The listing builds one solid part. Answer for the finished solid, in the listing's coordinates (mm). A direction names the side the tool comes from. Round coordinates to 2 decimals unless told otherwise and drop trailing zeros. Write each loop counter-clockwise with the first axis right and the second up, starting at its lowest first coordinate (ties: lowest second). Pieces come first, ordered by that corner, then holes. Notation, with made-up numbers: M 27,-12 L 48,-12 A24 cw 48,26 Z; hole C 5,68.25 d5. An arc over 180 degrees is marked long. Put each result on its own line as item: value. Start each with the question number.
```python
from build123d import *

# Parameters (mm, degrees)
F0_R     = 6.35
F1_DEPTH = 50.8
F2_R     = 44.45
F3_DEPTH = 127
F4_R     = 5.08
F5_R     = 5.08
F7_DEPTH = 12.7


with BuildPart() as f1:
    # F0 (on Front) → F1 (new body)
    with BuildSketch(Plane.XZ):
        Circle(F0_R)
    extrude(amount=F1_DEPTH)

    # F2 (on face) → F3 (join)
    with BuildSketch(Plane.XZ.offset(50.8)):
        Circle(F2_R)
    extrude(amount=F3_DEPTH)

    # F4
    f4_edges = [f1.edges().sort_by_distance(p)[0] for p in [
        (-44.45, -50.8, 0),
    ]]
    fillet(f4_edges, radius=F4_R)

    # F5
    f5_edges = [f1.edges().sort_by_distance(p)[0] for p in [
        (-44.45, -177.8, 0),
    ]]
    fillet(f5_edges, radius=F5_R)

    # F6 (on face) → F7 (cut)
    with BuildSketch(Plane(origin=(0, 0, 0), x_dir=(-1, 0, 0), z_dir=(0, 1, 0))):
        with BuildLine():
            ThreePointArc((0, 6.35), (-0.6382319087, 6.3178445716), (-1.27, 6.2217039467))
            Line((-1.27, 6.2217039467), (-1.27, 3.81))
            Line((-1.27, 3.81), (0, 3.81))
            Line((0, 3.81), (0, 6.35))
        make_face()
        with BuildLine():
            Line((1.27, 3.81), (1.27, 6.2217039467))
            ThreePointArc((1.27, 6.2217039467), (0.6382319087, 6.3178445716), (0, 6.35))
            Line((0, 6.35), (0, 3.81))
            Line((0, 3.81), (1.27, 3.81))
        make_face()
    extrude(amount=-F7_DEPTH, mode=Mode.SUBTRACT)


solid = f1.part
```
Item 1: Flat-ended cylindrical pins translate along their axes: pin 1 (1.3 mm diameter, centred on x = 0.5, z = 4.5, fed in from +Y); pin 2 (1.9 mm diameter, centred on y = -4.5, z = 5.5, fed in from -X); pin 3 (5 mm diameter, centred on x = 8.5, y = -132, fed in from -Z). Find the tip coordinate at first contact, or state that the pin passes through.
Item 2: Section A-A (z = 0) is taken. Give the vertices of the cut face in (x, y), and give its area (3 significant figures).
Item 3: Section B-B (y = -127) is taken. Give the vertices of the cut face in (x, z), and give its area (3 significant figures).
Item 4: Consider line 1 along Z through (x, y) = (0.5, -139.5); line 2 along Y through (x, z) = (-19, -33); line 3 along Z through (x, y) = (1, -44.5). Determine where each line is inside the solid, lowest interval first. Write a range as [from, to].
Item 5: Which of the six approach directions +Z, -Z, +X, -X, +Y, -Y give full straight-line access (tool end or side, diameter ignored) to faces 1 (the cylindrical face through (42.397, -113.482, 13.352)), 2 (the cylindrical face through (-1.38, -25.04, -6.2))?
Output values:
1. pin 1: stops at y = -12.7
1. pin 2: stops at x = -4.43
1. pin 3: stops at z = -44.04
2. outline: M -44.45,-172.72 A5.08 ccw -39.37,-177.8 L 39.37,-177.8 A5.08 ccw 44.45,-172.72 L 44.45,-55.88 A5.08 ccw 39.37,-50.8 L 6.35,-50.8 L 6.35,0 L -6.35,0 L -6.35,-50.8 L -39.37,-50.8 A5.08 ccw -44.45,-55.88 Z
2. area: 11,900 mm^2
3. outline: C 0,0 d88.9
3. area: 6,210 mm^2
4. line 1: z = [-44.45, 44.45]
4. line 2: y = [-177.8, -50.8]
4. line 3: z = [-6.27, 6.27]
5. face 1: +Y, -Y
5. face 2: +Y
